from build123d import *

# Parameters (mm, degrees)
SKETCH_W             = 20
SKETCH_H             = 40
PAD_DEPTH            = 60
SKETCH001_R          = 1.55
POCKET_DEPTH         = 6
SKETCH002_R          = 1.55
POCKET001_DEPTH      = 6
SKETCH004_R          = 1.55
POCKET003_DEPTH      = 8
SKETCH005_R          = 20
SKETCH005_R_2        = 2.55
POCKET004_DEPTH      = 20
SKETCH013_R          = 1.55
POCKET011_DEPTH      = 53.206
POCKET011_DEPTH_BACK = 53.206
SKETCH014_R          = 3
POCKET012_DEPTH      = 31.206
SKETCH015_R          = 3
POCKET013_DEPTH      = 31.206
FILLET_R             = 2


with BuildPart() as part:
    # Sketch → Pad (new body)
    with BuildSketch(Plane.XY):
        with BuildLine():
            Line((-53.205, 0), (-16.535, 63.5143031136))
            Line((-16.535, 63.5143031136), (-33.8555080757, 73.5143031136))
            Line((-33.8555080757, 73.5143031136), (-21.7278633238, 94.52))
            ThreePointArc((-13.0676092859, 99.52), (-18.0676092859, 98.1802540378), (-21.7278633238, 94.52))
            Line((-13.0676092859, 99.52), (13.0676092859, 99.52))
            ThreePointArc((21.7278633238, 94.52), (18.0676092859, 98.1802540378), (13.0676092859, 99.52))
            Line((33.8555080757, 73.5143031136), (21.7278633238, 94.52))
            Line((16.535, 63.5143031136), (33.8555080757, 73.5143031136))
            Line((53.205, 0), (16.535, 63.5143031136))
            Line((53.205, 0), (48.0088475773, -3))
            Line((48.0088475773, -3), (40.9247597743, 9.27))
            ThreePointArc((40.9247597743, 9.27), (39.0946327554, 11.1001270189), (36.5946327554, 11.77))
            Line((-36.5946327554, 11.77), (36.5946327554, 11.77))
            ThreePointArc((-36.5946327554, 11.77), (-39.0946327554, 11.1001270189), (-40.9247597743, 9.27))
            Line((-48.0088475773, -3), (-40.9247597743, 9.27))
            Line((-53.205, 0), (-48.0088475773, -3))
        make_face()
        with Locations((0, 73.52)):
            Rectangle(SKETCH_W, SKETCH_H, mode=Mode.SUBTRACT)
        with BuildLine():
            Line((-22.305213593, 41.52), (-34.2852316787, 20.77))
            ThreePointArc((-34.2852316787, 20.77), (-34.2852316787, 18.77), (-32.5531808711, 17.77))
            Line((-32.5531808711, 17.77), (32.5531808711, 17.77))
            ThreePointArc((32.5531808711, 17.77), (34.2852316787, 18.77), (34.2852316787, 20.77))
            Line((34.2852316787, 20.77), (22.305213593, 41.52))
            ThreePointArc((22.305213593, 41.52), (19.3770103627, 44.4482032303), (15.3770103627, 45.52))
            Line((15.3770103627, 45.52), (-15.3770103627, 45.52))
            ThreePointArc((-15.3770103627, 45.52), (-19.3770103627, 44.4482032303), (-22.305213593, 41.52))
        make_face(mode=Mode.SUBTRACT)
    extrude(amount=PAD_DEPTH)

    # Sketch001 (on DatumPlane) → Pocket (cut, symmetric)
    with BuildSketch(Plane(origin=(53, 0, 0), x_dir=(-0.5, 0.8660254038, 0), z_dir=(0.8660254038, 0.5, 0))):
        with Locations((47.2375, 50)):
            Circle(SKETCH001_R)
        with Locations((9.8975, 50)):
            Circle(SKETCH001_R)
        with Locations((47.2375, 10)):
            Circle(SKETCH001_R)
        with Locations((9.8975, 10)):
            Circle(SKETCH001_R)
    extrude(amount=POCKET_DEPTH, both=True, mode=Mode.SUBTRACT)

    # Sketch002 (on DatumPlane) → Pocket001 (cut, symmetric)
    with BuildSketch(Plane(origin=(-53, 0, 0), x_dir=(0.5, 0.8660254038, 0), z_dir=(0.8660254038, -0.5, 0))):
        with Locations((47.2375, 50)):
            Circle(SKETCH002_R)
        with Locations((47.2375, 10)):
            Circle(SKETCH002_R)
        with Locations((9.8975, 10)):
            Circle(SKETCH002_R)
        with Locations((9.8975, 50)):
            Circle(SKETCH002_R)
    extrude(amount=POCKET001_DEPTH, both=True, mode=Mode.SUBTRACT)

    # Sketch004 → Pocket003 (cut)
    with BuildSketch(Plane(origin=(0, 99.52, 0), x_dir=(-1, 0, 0), z_dir=(0, 1, 0))):
        with Locations((0, 50)):
            Circle(SKETCH004_R)
        with Locations((0, 10)):
            Circle(SKETCH004_R)
    extrude(amount=-POCKET003_DEPTH, mode=Mode.SUBTRACT)

    # Sketch005 → Pocket004 (cut)
    with BuildSketch(Plane.XZ):
        with Locations((0, 30)):
            Circle(SKETCH005_R)
        with Locations((23.5, 53.5)):
            Circle(SKETCH005_R_2)
        with Locations((23.5, 6.5)):
            Circle(SKETCH005_R_2)
        with Locations((-23.5, 6.5)):
            Circle(SKETCH005_R_2)
        with Locations((-23.5, 53.5)):
            Circle(SKETCH005_R_2)
    extrude(amount=-POCKET004_DEPTH, mode=Mode.SUBTRACT)

    # Sketch013 → Pocket011 (cut, two sides)
    with BuildSketch(Plane.YZ) as pocket011_sk:
        with Locations((83.52, 50)):
            Circle(SKETCH013_R)
        with Locations((83.52, 10)):
            Circle(SKETCH013_R)
    extrude(amount=-POCKET011_DEPTH, mode=Mode.SUBTRACT)
    extrude(pocket011_sk.sketch, amount=POCKET011_DEPTH_BACK, mode=Mode.SUBTRACT)

    # Sketch014 → Pocket012 (cut, through all)
    with BuildSketch(Plane.YZ.offset(22)):
        with Locations((83.52, 50)):
            Circle(SKETCH014_R)
        with Locations((83.52, 10)):
            Circle(SKETCH014_R)
    extrude(amount=POCKET012_DEPTH, mode=Mode.SUBTRACT)

    # Sketch015 → Pocket013 (cut, through all)
    with BuildSketch(Plane.YZ.offset(-22)):
        with Locations((83.52, 50)):
            Circle(SKETCH015_R)
        with Locations((83.52, 10)):
            Circle(SKETCH015_R)
    extrude(amount=-POCKET013_DEPTH, mode=Mode.SUBTRACT)

    # Fillet
    fillet_edges = [part.edges().sort_by_distance(p)[0] for p in [
        (27.791686, 84.017152, 60),
        (18.067609, 98.180254, 60),
        (0, 99.52, 60),
        (-18.067609, 98.180254, 60),
        (-27.791686, 84.017152, 60),
        (27.791686, 84.017152, 0),
        (18.067609, 98.180254, 0),
        (0, 99.52, 0),
        (-18.067609, 98.180254, 0),
        (-27.791686, 84.017152, 0),
    ]]
    fillet(fillet_edges, radius=FILLET_R)


solid = part.part
Can you work these out from the model? Positions are in its coordinate system, mm. A direction names the side the tool comes from. Give positions to 0.01 mm unless a question says otherwise; leave off trailing zeros. Loops run counter-clockwise (first coordinate to the right, second up) from the corner with the lowest first, then second, coordinate; pieces in that order, holes last. Notation, with made-up numbers: (4.5, 41.5) - (11.5, 41.5) arc R30 cw to (11.5, 64.5) - close; hole circle Ø3 at (51.5, 20.5). An arc over 180 degrees is marked (long way). One line per item, written item: value.
(1) I'm going to push flat-ended pins straight in: pin 1 (4 mm diameter, centred on x = 23.5, z = 6.5, fed in from -Y); pin 2 (4 mm diameter, centred on y = 82.5, z = 10.5, fed in from +X); pin 3 (2 mm diameter, centred on y = 87.5, z = 43.5, fed in from +X); pin 4 (1.9 mm diameter, centred on y = 83.52, z = 50, fed in from +X). Where does each tip first touch, or does it pass through?
Verdict:
pin 1: y = 35.99
pin 2: x = 29.82
pin 3: x = 26.36
pin 4: through
(2) If we mould it in two halves opening along Y, with no side actions, what happens to faces 1 (the face through (-50.64, -1.48, 29.58)), 2 (the face through (-27.877, 83.87, 29.608)), 3 (the face through (-26, 15, 7)), 4 (the face through (0, 53.52, 30))? For each: released by +Y, released by -Y, zero draft, split by the parting line, or undercut.
Verdict:
face 1: released by -Y
face 2: released by +Y
face 3: zero draft
face 4: undercut
(3) If we section it at C-C, the plane y = 31: List the corners of the cut face in (x, z) for me.
Verdict:
outline: (-35.31, 0) - (-28.38, 0) - (-28.38, 60) - (-35.31, 60) - close; (28.38, 0) - (35.31, 0) - (35.31, 60) - (28.38, 60) - close
(4) On a 3-axis mill with a long thin cutter (end or side, diameter ignored), from which of +Z, -Z, +X, -X, +Y, -Y can I reach the whole of each face in a straight line? I mean faces 5 (the face through (4, 47, 0)), 6 (the face through (0, 93.52, 30)), 7 (the face through (-2.6, 14.73, 49.83)), 8 (the face through (-35.13, 31.31, 29.58)), 9 (the face through (-45.739, 6.848, 48.487)). Say none if no direction works.
Verdict:
face 5: -Z, +X, -X, +Y, -Y
face 6: +Z, -Z
face 7: -Y
face 8: +Z, -Z, -X
face 9: none
(5) If we section it at B-B, the plane x = -6.5: List the corners of the cut face in (y, z) for me.
Verdict:
outline: (11.77, 0) - (17.77, 0) - (17.77, 11.09) - (11.77, 11.09) - close; (11.77, 48.91) - (17.77, 48.91) - (17.77, 60) - (11.77, 60) - close; (45.52, 0) - (53.52, 0) - (53.52, 60) - (45.52, 60) - close; (93.52, 0) - (97.52, 0) arc R2 ccw to (99.52, 2) - (99.52, 58) arc R2 ccw to (97.52, 60) - (93.52, 60) - close
(6) I need wall thicknesses on line 1 along Y through (x, z) = (-4, 52.5); line 2 along Z through (x, y) = (0, 95.9); line 3 along Y through (x, z) = (21.5, 48). Which ranges of each line are inside material? Lowest first, please.
Verdict:
line 1: 11.77 to 17.77, 45.52 to 53.52, 93.52 to 99.52
line 2: 0 to 8.45, 11.55 to 48.45, 51.55 to 60
line 3: 11.77 to 17.77, 42.67 to 54.91, 66.38 to 94.9
